from build123d import *

# Parameters (mm, degrees)
SKETCH_1_W               = 60
SKETCH_1_H               = 60
EXTRUDE_1_DEPTH          = 15
SKETCH_2_W               = 20
SKETCH_2_H               = 60
EXTRUDE_2_DEPTH          = 13
SKETCH_3_W               = 15
SKETCH_3_H               = 15
CUT_EXTRUDE_1_DEPTH      = 51.833060109
SKETCH_5_R               = 4
CUT_EXTRUDE_3_DEPTH      = 51.833060109
MIRROR_2_COPY_1_SKETCH_R = 4
MIRROR_2_COPY_1_DEPTH    = 51.833060109


with BuildPart() as part:
    # Эскиз1 → Бобышка-Вытянуть1 (new body)
    with BuildSketch(Plane.XY):
        Rectangle(SKETCH_1_W, SKETCH_1_H)
    extrude(amount=EXTRUDE_1_DEPTH)

    # Эскиз2 → Бобышка-Вытянуть2 (add)
    with BuildSketch(Plane.XY.offset(15)):
        Rectangle(SKETCH_2_W, SKETCH_2_H)
    extrude(amount=EXTRUDE_2_DEPTH)

    # Эскиз3 → Вырез-Вытянуть1 (cut, through all)
    with BuildSketch(Plane.XY.offset(28)):
        Rectangle(SKETCH_3_W, SKETCH_3_H)
    extrude(amount=-CUT_EXTRUDE_1_DEPTH, mode=Mode.SUBTRACT)

    # Эскиз5 → Вырез-Вытянуть3 (cut, through all)
    with BuildSketch(Plane(origin=(0, 0, 0), x_dir=(-1, 0, 0), z_dir=(0, 0, -1))):
        with Locations((-22.5, -22.5)):
            Circle(SKETCH_5_R)
    cut_extrude_3 = extrude(amount=-CUT_EXTRUDE_3_DEPTH, mode=Mode.SUBTRACT)

    # Зеркальное отражение1: Вырез-Вытянуть3 across plane
    add(cut_extrude_3.mirror(Plane.ZX), mode=Mode.SUBTRACT)

    # Зеркальное отражение2: Вырез-Вытянуть3 across plane
    add(cut_extrude_3.mirror(Plane(origin=(0, 0, 0), x_dir=(0, 0, 1), z_dir=(1, 0, 0))), mode=Mode.SUBTRACT)

    # Зеркальное отражение2 copy 1 sketch → Зеркальное отражение2 copy 1 (cut, through all)
    with BuildSketch(Plane(origin=(0, 0, 0), x_dir=(1, 0, 0), z_dir=(0, 0, -1))):
        with Locations((-22.5, -22.5)):
            Circle(MIRROR_2_COPY_1_SKETCH_R)
    extrude(amount=-MIRROR_2_COPY_1_DEPTH, mode=Mode.SUBTRACT)


solid = part.part
The model under review builds one solid part; all positions refer to its coordinate system, in mm. A direction names the side the tool comes from. Round coordinates to 2 decimals unless told otherwise and drop trailing zeros. Write each loop counter-clockwise with the first axis right and the second up, starting at its lowest first coordinate (ties: lowest second). Pieces come first, ordered by that corner, then holes. Notation, with made-up numbers: (80, 55) -> (109, 55) arc R24 cw to (109, 74) -> close; hole circle Ø6 at (74.5, 58.5). An arc over 180 degrees is marked (long way). Answer as a JSON object with one key per item and string values.
1. We need section C-C on x = 22.5. State the section outline as (y, z) points, and give its area (3 significant figures).
Results found:
{"outline": "(-30, 0) -> (-26.5, 0) -> (-26.5, 15) -> (-30, 15) -> close; (-18.5, 0) -> (18.5, 0) -> (18.5, 15) -> (-18.5, 15) -> close; (26.5, 0) -> (30, 0) -> (30, 15) -> (26.5, 15) -> close", "area": "660 mm^2"}
2. We need section A-A on x = 6.5. State the section outline as (y, z) points, and give its area (3 significant figures).
Results found:
{"outline": "(-30, 0) -> (-7.5, 0) -> (-7.5, 28) -> (-30, 28) -> close; (7.5, 0) -> (30, 0) -> (30, 28) -> (7.5, 28) -> close", "area": "1,260 mm^2"}
3. Machinability: for faces 5 (the face through (7.5, 0, 14)), 6 (the face through (20, 0, 15)), 7 (the face through (-20, 0, 15)), which of the approach directions +Z, -Z, +X, -X, +Y, -Y give a long, thin tool a straight path to every point of the face, cutting with its end or side? Answer none if there is none.
Results found:
{"face 5": "+Z, -Z", "face 6": "+Z, +X, +Y, -Y", "face 7": "+Z, -X, +Y, -Y"}
4. To check wall thickness, follow line 1 along X through (y, z) = (22.5, 4.75); line 2 along Y through (x, z) = (2.5, 14.5). State the ranges of each line that lie inside material, in increasing order.
Results found:
{"line 1": "x = -30 to -26.5, -18.5 to 18.5, 26.5 to 30", "line 2": "y = -30 to -7.5, 7.5 to 30"}
5. The part is to be moulded in two halves that separate along Y. For faces 1 (the face through (0, 30, 11)), 2 (the face through (-10, 0, 21)), 3 (the face through (0, -30, 11)), 4 (the face through (0, -7.5, 14)), say which applies: pulls with the +Y half, pulls with the -Y half, needs draft (parallel to the pull), parting line crosses it, or undercut.
Results found:
{"face 1": "pulls with the +Y half", "face 2": "needs draft", "face 3": "pulls with the -Y half", "face 4": "undercut"}
6. Clearance check with flat-ended pins moving along their axes: pin 1 (10.5 mm diameter, centred on y = 0, z = 22, fed in from +X); pin 2 (16 mm diameter, centred on x = -21, y = -14, fed in from +Z); pin 3 (4 mm diameter, centred on y = 8, z = 21, fed in from -X). State where each tip first meets the part, or that it passes through.
Results found:
{"pin 1": "stops at x = 10", "pin 2": "stops at z = 15", "pin 3": "stops at x = -10"}
7. We need section D-D on z = 4. State the section outline as (x, y) points.
Results found:
{"outline": "(-30, -30) -> (30, -30) -> (30, 30) -> (-30, 30) -> close; hole circle Ø8 at (-22.5, -22.5); hole circle Ø8 at (-22.5, 22.5); hole (-7.5, -7.5) -> (7.5, -7.5) -> (7.5, 7.5) -> (-7.5, 7.5) -> close; hole circle Ø8 at (22.5, -22.5); hole circle Ø8 at (22.5, 22.5)"}
8. We need section B-B on y = 1.5. State the section outline as (x, z) points.
Results found:
{"outline": "(-30, 0) -> (-7.5, 0) -> (-7.5, 28) -> (-10, 28) -> (-10, 15) -> (-30, 15) -> close; (7.5, 0) -> (30, 0) -> (30, 15) -> (10, 15) -> (10, 28) -> (7.5, 28) -> close"}
